Autodesk Inventor part; units mm, degrees
ref_plane "YZ Plane" through (0, 0, 0) normal (1, 0, 0) x (0, 1, 0)
ref_plane "XZ Plane" through (0, 0, 0) normal (0, 1, 0) x (-1, 0, 0)
ref_plane "XY Plane" through (0, 0, 0) normal (0, 0, 1) x (1, 0, 0)
sketch "Sketch1" plane through (0, 0, 0) normal (0, 1, 0) x (-1, 0, 0)
  line L0 (-0.75, -1.6) -> (0.75, -1.6)
  line L1 (0.75, -1.6) -> (0.75, 1.6)
  line L2 (0.75, 1.6) -> (-0.75, 1.6)
  line L3 (-0.75, 1.6) -> (-0.75, -1.6)
  line L4 (-0.75, -1.6) -> (0.75, 1.6) construction
  line L5 (0.75, -1.6) -> (-0.75, 1.6) construction
  line L6 (0.75, 1.6) -> (-0.75, 1.6)
  line L7 (-0.75, 1.6) -> (-0.75, 2.6)
  line L8 (-0.75, 2.6) -> (0.75, 2.6)
  line L9 (0.75, 2.6) -> (0.75, 1.6)
  line L10 (-0.75, -1.6) -> (0.75, -1.6)
  line L11 (0.75, -1.6) -> (0.75, -2.6)
  line L12 (0.75, -2.6) -> (-0.75, -2.6)
  line L13 (-0.75, -2.6) -> (-0.75, -1.6)
  point P0 (0, 0)
  point P1 (0.75, -1.6)
  dimension "d0" = 3.2
  dimension "d1" = 1.5
  dimension "d2" = 1
  dimension "d3" = 1
extrude "Extrusion1" add sketch "Sketch1" along normal blind 0.5 contours L0 L11 L12 L13 | L7 L8 L9 L2
sketch "Sketch2" plane through (0.75, 0, 2.6) normal (1, 0, 0) x (0, 0, -1)
  line L0 (0, 0.5) -> (1, 0.5)
  line L1 (0.85, 0.5) -> (4.35, 0.5)
  line L2 (4.35, 0.5) -> (4.35, 1.5)
  line L3 (4.35, 1.5) -> (0.85, 1.5)
  line L4 (0.85, 1.5) -> (0.85, 0.5)
  line L5 (0.85, 1.5) -> (0, 0.5)
  line L6 (5.2, 0) -> (5.2, 0.5)
  line L7 (4.35, 1.5) -> (5.2, 0.5)
  line L8 (0, 0) -> (1, 0) construction
  line L9 (0, 0) -> (5.2, 0) construction
  line L10 (2.6, 0) -> (2.6, 2.5684) construction
  line L11 (0, 0.5) -> (5.2, 0.5)
  point P0 (2.6, 0.5)
  dimension "d10" = 3.5
  dimension "d19" = 1
extrude "Extrusion3" add sketch "Sketch2" against normal blind 1.5
sketch "Sketch5" plane through (0.75, 1.5, 1.75) normal (0, 1, 0) x (1, 0, 0)
  line L0 (-1.5, 0) -> (-1.5, 3.5)
  line L1 (0, 3.5) -> (0, 0)
  line L2 (-1.5, 3.5) -> (0, 3.5)
  line L3 (0, 3.5) -> (0, 0)
  line L4 (0, 0) -> (-1.5, 0)
  line L5 (-1.5, 0) -> (-1.5, 3.5)
  point P0 (-0.75, 1.75)
  point P1 (0, 3.5)
  point P2 (-1.5, 0)
extrude "Extrusion5" add sketch "Sketch5" along normal blind 2
sketch "Sketch6" plane through (0.75, 3.5, 1.75) normal (0, 1, 0) x (1, 0, 0)
  line L0 (-1.5, 3) -> (0, 3)
  line L1 (0, 3) -> (0, 0.5)
  line L2 (0, 0.5) -> (-1.5, 0.5)
  line L3 (-1.5, 0.5) -> (-1.5, 3)
  line L4 (0, 0) -> (0, 3.5) construction
  line L5 (0, 0) -> (0, 0.5) construction
  line L6 (-0.75, 3) -> (-0.75, 3.5) construction
  line L7 (0, 3.5) -> (-1.5, 3.5) construction
  line L8 (-0.75, 0.5) -> (-0.75, 0) construction
  point P0 (-0.75, 1.75)
  point P1 (-1.5, 1.75)
  point P2 (0, 1.75)
  dimension "d20" = 2.5
extrude "Extrusion6" add sketch "Sketch6" along normal blind 5.5
fillet "Fillet1" radius 0.6 4 edges at (0, 9, -1.25) (-0.75, 9, 0) (0, 9, 1.25) (0.75, 9, 0)
sketch "Sketch7" plane through (0, 0, 0) normal (0, -1, 0) x (1, 0, 0)
  line L0 (-0.75, 2.6) -> (0.75, 2.6)
  line L1 (-0.75, -2.6) -> (0.75, -2.6)
  line L2 (0.75, -2.6) -> (0.75, 2.6)
  line L3 (0.75, 2.6) -> (-0.75, 2.6)
  line L4 (-0.75, 2.6) -> (-0.75, -2.6)
  line L5 (-0.75, -2.6) -> (0.75, 2.6) construction
  line L6 (0.75, -2.6) -> (-0.75, 2.6) construction
  point P0 (0, 0)
sketch "Sketch8" plane through (0.75, 0.5, -2.6) normal (0, -1, 0) x (1, 0, 0)
  line L0 (-1.5, 5.2) -> (0, 5.2)
  line L1 (0, 4.35) -> (-1.5, 4.35)
  line L2 (0, 5.2) -> (-1.5, 5.2)
  line L3 (-1.5, 5.2) -> (-1.5, 4.35)
  line L4 (-1.5, 4.35) -> (0, 4.35)
  line L5 (0, 4.35) -> (0, 5.2)
  line L6 (0, 0) -> (-1.5, 0)
  line L7 (0, 0.85) -> (-1.5, 0.85)
  line L8 (0, 0) -> (-1.5, 0)
  line L9 (-1.5, 0) -> (-1.5, 0.85)
  line L10 (-1.5, 0.85) -> (0, 0.85)
  line L11 (0, 0.85) -> (0, 0)
  point P0 (-0.75, 2.6)
  point P1 (0, 0.85)
sketch "Sketch4" plane through (0.75, 1.5, 1.75) normal (0, 1, 0) x (1, 0, 0)
  line L0 (-1.5, 3) -> (0, 3)
  line L1 (0, 3) -> (0, 0.5)
  line L2 (0, 0.5) -> (-1.5, 0.5)
  line L3 (-1.5, 0.5) -> (-1.5, 3)
  line L4 (-1.5, 0) -> (-1.5, 3.5)
  line L5 (0, 3.5) -> (0, 0)
  line L6 (0, 3.5) -> (-1.5, 3.5)
  point P0 (-0.75, 1.75)
  point P1 (-1.5, 1.75)
  point P2 (0, 1.75)
  point P3 (-0.75, 3)
  dimension "d13" = 2.5
  dimension "d14" = 0.5
properties part number "LightPipe"
Can you work these out from the model? Positions are in its coordinate system, mm. A direction names the side the tool comes from. Round coordinates to 2 decimals unless told otherwise and drop trailing zeros. Write each loop counter-clockwise with the first axis right and the second up, starting at its lowest first coordinate (ties: lowest second). Pieces come first, ordered by that corner, then holes. Notation, with made-up numbers: M 80.5,-16.75 L 133.5,-16.75 A28 ccw 133.5,11.25 Z; hole C -28.5,71.5 d3. An arc over 180 degrees is marked long. Use a Markdown table: item, result.
Item 1: I want a section at A-A (y = 2.75). List the corners of the cut face in (x, z) for me.
Found:
| item | result |
|---|---|
| outline | M -0.75,-1.75 L 0.75,-1.75 L 0.75,1.75 L -0.75,1.75 Z |
Item 2: If I drill on line 1 along Y through (x, z) = (0.5, -1.45); line 2 along Z through (x, y) = (-0.55, 4); line 3 along Y through (x, z) = (0, 0.1), over which ranges is the centre line in solid material (lowest first)? Write a range as [from, to].
Found:
| item | result |
|---|---|
| line 1 | y = [0.5, 3.5] |
| line 2 | z = [-1.25, 1.25] |
| line 3 | y = [0.5, 9] |
Item 3: Which directions (+Z, -Z, +X, -X, +Y, -Y) give clear straight access to the entire face, cutting with the end or side of a thin tool? Please do faces 1 (the face through (0, 6, 1.25)), 2 (the face through (0, 6, -1.25)), 3 (the face through (0, 0.5, 0)).
Found:
| item | result |
|---|---|
| face 1 | +Z, +X, -X, +Y |
| face 2 | -Z, +X, -X, +Y |
| face 3 | +X, -X, -Y |
Item 4: I want a section at C-C (x = -0.25). List the corners of the cut face in (y, z) for me, and give its area (3 significant figures).
Found:
| item | result |
|---|---|
| outline | M 0,-2.6 L 0.5,-2.6 L 1.5,-1.75 L 3.5,-1.75 L 3.5,-1.25 L 8.4,-1.25 A0.6 ccw 8.99,-0.75 L 8.99,0.75 A0.6 ccw 8.4,1.25 L 3.5,1.25 L 3.5,1.75 L 1.5,1.75 L 0.5,2.6 L 0,2.6 L 0,1.6 L 0.5,1.6 L 0.5,-1.6 L 0,-1.6 Z |
| area | 25.9 mm2 |
Item 5: I want a section at B-B (z = -0.25). List the corners of the cut face in (x, y) for me.
Found:
| item | result |
|---|---|
| outline | M -0.75,0.5 L 0.75,0.5 L 0.75,8.4 A0.6 ccw 0.15,9 L -0.15,9 A0.6 ccw -0.75,8.4 Z |
Item 6: I want a section at D-D (x = 0.3). List the corners of the cut face in (y, z) for me, and give its area (3 significant figures).
Found:
| item | result |
|---|---|
| outline | M 0,-2.6 L 0.5,-2.6 L 1.5,-1.75 L 3.5,-1.75 L 3.5,-1.25 L 8.4,-1.25 A0.6 ccw 8.98,-0.8 L 8.98,0.8 A0.6 ccw 8.4,1.25 L 3.5,1.25 L 3.5,1.75 L 1.5,1.75 L 0.5,2.6 L 0,2.6 L 0,1.6 L 0.5,1.6 L 0.5,-1.6 L 0,-1.6 Z |
| area | 25.9 mm2 |
Item 7: For pin 1 Ø0.8 at (x, y) = (0, 2) entering from -Z, with a flat end and sliding along its axis, tell me the tip position at first contact or that it passes through.
Found:
| item | result |
|---|---|
| pin 1 | stops at z = -1.75 |
